Check sheet for the modelled part. Datum: model origin and axes. Units: mm. Face numbers are marked on the shaded views. A direction names the side the tool comes from. Coordinates: 2 decimals unless noted, no trailing zeros. Loops run counter-clockwise (first coordinate to the right, second up) from the corner with the lowest first, then second, coordinate; pieces in that order, holes last. Notation, with made-up numbers: (63, 46) -> (83, 46) arc R24 cw to (83, 67) -> close; hole circle Ø7 at (-21, 87). An arc over 180 degrees is marked (long way). Use one line per item in the form item = value.
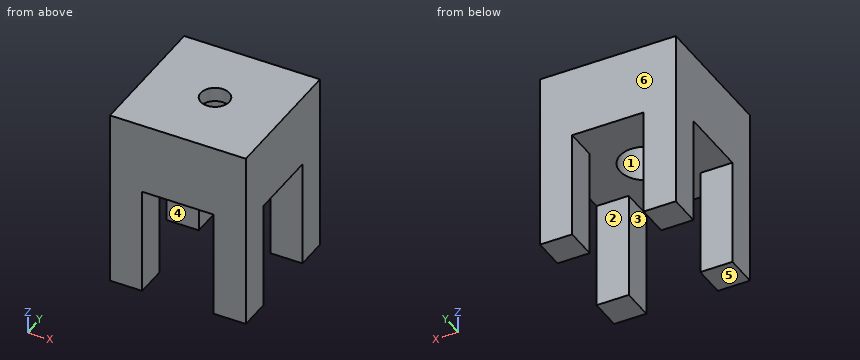
from build123d import *

# Parameters (mm, degrees)
F0_W           = 19
F0_H           = 5
F1_DEPTH       = 9.5
F2_DEPTH       = 9.5
F3_W           = 10
F3_H           = 15
F4_DEPTH       = 25
F6_D           = 4
F6_CBORE_D     = 7
F6_CBORE_DEPTH = 8


with BuildPart() as f1:
    # F0 (on Front) → F1 (new body, symmetric)
    with BuildSketch(Plane.XZ):
        with Locations((-7.338427, -8.679005)):
            Rectangle(F0_W, F0_H)
    extrude(amount=F1_DEPTH, both=True)

    # F0 (on Front) → F2 (join, symmetric)
    with BuildSketch(Plane.XZ):
        Polygon((2.161573, -31.179005), (2.161573, -11.179005), (-16.838427, -11.179005), (-16.838427, -31.179005), (-12.338427, -31.179005), (-12.338427, -16.179005), (-2.338427, -16.179005), (-2.338427, -31.179005), align=None)
    extrude(amount=F2_DEPTH, both=True)

    # F3 (on face) → F4 (cut)
    with BuildSketch(Plane(origin=(-16.838427, 0, 0), x_dir=(0, -1, 0), z_dir=(-1, 0, 0))):
        with Locations((0, -23.679005)):
            Rectangle(F3_W, F3_H)
    extrude(amount=-F4_DEPTH, mode=Mode.SUBTRACT)

    # F6 (through all)
    with Locations(Plane(origin=(0, 0, -16.179005), x_dir=(1, 0, 0), z_dir=(0, 0, -1))):
        with Locations((-7.338427, 0)):
            CounterBoreHole(F6_D / 2, F6_CBORE_D / 2, F6_CBORE_DEPTH)


solid = f1.part
(1) Section check D-D, the plane y = 5.75. Record the boundary of the cut face in (x, z), plus the area to 3 significant figures.
Established:
outline = (-16.84, -31.18) -> (-12.34, -31.18) -> (-12.34, -16.18) -> (-2.34, -16.18) -> (-2.34, -31.18) -> (2.16, -31.18) -> (2.16, -6.18) -> (-16.84, -6.18) -> close
area = 325 mm²
(2) Go/stop test with flat-tipped pins: P1, Ø3, axis at x = -12, y = 1, coming from the -Z side; P2, Ø2, axis at x = -8, y = -1.5, coming from the -Z side. Record where each tip stops, or that it passes through.
Established:
P1 = -16.18
P2 = -8.18
(3) Mould release check, pull along Y, two halves, no side actions. Record for the marked faces 4, 5 and 6: +Y half, -Y half, draft (parallel to the pull), parting line (faces both ways), or undercut.
Established:
face_4 = undercut
face_5 = draft
face_6 = +Y half
(4) Scan lines: line 1 along X through (y, z) = (-8, -28.5); line 2 along Z through (x, y) = (-3, -7.5); line 3 along Z through (x, y) = (-8.5, -2.25). Record each from-to range of solid material in increasing order.
Established:
line_1 = -16.84 to -12.34, -2.34 to 2.16
line_2 = -16.18 to -6.18
line_3 = -8.18 to -6.18
(5) Tool access check on the marked faces 1, 2 and 3. Record the directions out of +Z, -Z, +X, -X, +Y, -Y that give a thin tool (end or side, any length) a straight path to the whole face; none if there is none.
Established:
face_1 = -Z
face_2 = -Z, +X, -X
face_3 = -Z, +Y, -Y
(6) Section check A-A, the plane z = -20. Record the boundary of the cut face in (x, y), plus the area to 3 significant figures.
Established:
outline = (-16.84, -9.5) -> (-12.34, -9.5) -> (-12.34, -5) -> (-16.84, -5) -> close; (-16.84, 5) -> (-12.34, 5) -> (-12.34, 9.5) -> (-16.84, 9.5) -> close; (-2.34, -9.5) -> (2.16, -9.5) -> (2.16, -5) -> (-2.34, -5) -> close; (-2.34, 5) -> (2.16, 5) -> (2.16, 9.5) -> (-2.34, 9.5) -> close
area = 81.0 mm²
(7) Section check B-B, the plane y = 0. Record the boundary of the cut face in (x, z), plus the area to 3 significant figures.
Established:
outline = (-16.84, -16.18) -> (-10.84, -16.18) -> (-10.84, -8.18) -> (-9.34, -8.18) -> (-9.34, -6.18) -> (-16.84, -6.18) -> close; (-5.34, -8.18) -> (-3.84, -8.18) -> (-3.84, -16.18) -> (2.16, -16.18) -> (2.16, -6.18) -> (-5.34, -6.18) -> close
area = 126 mm²
(8) Section check C-C, the plane x = -7.5. Record the boundary of the cut face in (y, z).
Established:
outline = (-9.5, -16.18) -> (-3.5, -16.18) -> (-3.5, -8.18) -> (-1.99, -8.18) -> (-1.99, -6.18) -> (-9.5, -6.18) -> close; (1.99, -8.18) -> (3.5, -8.18) -> (3.5, -16.18) -> (9.5, -16.18) -> (9.5, -6.18) -> (1.99, -6.18) -> close
